Build history of the part. All positions in model axes, mm. A direction names the side the tool comes from. Give positions to 0.01 mm unless a question says otherwise; leave off trailing zeros. Loops run counter-clockwise (first coordinate to the right, second up) from the corner with the lowest first, then second, coordinate; pieces in that order, holes last. Notation, with made-up numbers: (54.5, 23) -> (67.5, 23) arc R28 cw to (67.5, 53) -> close; hole circle Ø7 at (60.25, 21). An arc over 180 degrees is marked (long way). Answer as a JSON object with one key per item and string values. Group by question number.
from build123d import *

# Parameters (mm, degrees)
SKETCH1_R           = 1.75
BOSS_EXTRUDE1_DEPTH = 4
FILLET1_R           = 3


with BuildPart() as part:
    # Sketch1 → Boss-Extrude1 (new body)
    with BuildSketch(Plane(origin=(0, 0, 0), x_dir=(1, 0, 0), z_dir=(0, 1, 0))):
        with BuildLine():
            Line((20.877501001, 2.5), (3.122498999, 2.5))
            ThreePointArc((3.122498999, 2.5), (-4, 0), (3.122498999, -2.5))
            Line((3.122498999, -2.5), (20.877501001, -2.5))
            ThreePointArc((20.877501001, -2.5), (28, 0), (20.877501001, 2.5))
        make_face()
        Circle(SKETCH1_R, mode=Mode.SUBTRACT)
        with Locations((24, 0)):
            Circle(SKETCH1_R, mode=Mode.SUBTRACT)
    extrude(amount=BOSS_EXTRUDE1_DEPTH)

    # Fillet1
    fillet1_edges = [part.edges().sort_by_distance(p)[0] for p in [
        (20.877501001, 2, 2.5),
        (3.122498999, 2, 2.5),
        (3.122498999, 2, -2.5),
        (20.877501001, 2, -2.5),
    ]]
    fillet(fillet1_edges, radius=FILLET1_R)


solid = part.part
(1) 3-axis set-ups, long thin cutter, end or side, ignore diameter. For faces 3 (the cylindrical face through (-4, 2, 0)), 4 (the cylindrical face through (3.36, 2.03, -2.66)), 5 (the flat face through (12, 2, 2.5)): which of +Z, -Z, +X, -X, +Y, -Y reach the whole face in a straight line?
(2) Saw through at C-C on z = 0. List the corners of the cut face in (x, y), plus the area to 3 significant figures.
(3) Pin check, flat tips, straight feed: pin 1 (2 mm diameter, centred on y = 3, z = 2, fed in from -X); pin 2 (1 mm diameter, centred on x = 13.5, y = 2, fed in from -Z); pin 3 (1 mm diameter, centred on x = 2.5, y = 1.5, fed in from -Z). Stop position of each tip, or through.
(4) Pull direction X, two halves, no side cores. Call faces 1 (the flat face through (12, 0, 0)), 2 (the cylindrical face through (22.25, 1.97, -0.08)): pulls with the +X half, pulls with the -X half, needs draft (parallel to the pull), parting line crosses it, or undercut.
(5) Saw through at B-B on y = 3.3. List the corners of the cut face in (x, z), plus the area to 3 significant figures.
(6) Saw through at D-D on x = 0.5. List the corners of the cut face in (y, z), plus the area to 3 significant figures.
(7) Saw through at A-A on x = 24. List the corners of the cut face in (y, z), plus the area to 3 significant figures.
(8) Probe line 1 along X through (y, z) = (3.4, 1); line 2 along X through (y, z) = (3.45, 0.75); line 3 along Z through (x, y) = (14.5, 2.55). List the from-to ranges inside material, lowest first. Write a range as [from, to].
Calculated:
{
 "1": {"face 3": "+Y, -Y", "face 4": "-Z, +Y, -Y", "face 5": "+Z, +Y, -Y"},
 "2": {"outline": "(-4, 0) -> (-1.75, 0) -> (-1.75, 4) -> (-4, 4) -> close; (1.75, 0) -> (22.25, 0) -> (22.25, 4) -> (1.75, 4) -> close; (25.75, 0) -> (28, 0) -> (28, 4) -> (25.75, 4) -> close", "area": "100 mm^2"},
 "3": {"pin 1": "stops at x = -3.87", "pin 2": "stops at z = -2.5", "pin 3": "stops at z = -3.46"},
 "4": {"face 1": "needs draft", "face 2": "undercut"},
 "5": {"outline": "(2.47, -3.14) arc R3 cw to (4.33, -2.5) -> (19.67, -2.5) arc R3 cw to (21.53, -3.14) arc R4 ccw (long way) to (21.53, 3.14) arc R3 cw to (19.67, 2.5) -> (4.33, 2.5) arc R3 cw to (2.47, 3.14) arc R4 ccw (long way) to start; hole circle Ø3.5 at (0, 0); hole circle Ø3.5 at (24, 0)", "area": "165 mm^2"},
 "6": {"outline": "(0, -3.97) -> (4, -3.97) -> (4, -1.68) -> (0, -1.68) -> close; (0, 1.68) -> (4, 1.68) -> (4, 3.97) -> (0, 3.97) -> close", "area": "18.3 mm^2"},
 "7": {"outline": "(0, -4) -> (4, -4) -> (4, -1.75) -> (0, -1.75) -> close; (0, 1.75) -> (4, 1.75) -> (4, 4) -> (0, 4) -> close", "area": "18.0 mm^2"},
 "8": {"line 1": "x = [-3.87, -1.44], [1.44, 22.56], [25.44, 27.87]", "line 2": "x = [-3.93, -1.58], [1.58, 22.42], [25.58, 27.93]", "line 3": "z = [-2.5, 2.5]"}
}
